Geometry: final body of the model. Coordinates: model frame, mm. A direction names the side the tool comes from. Give positions to 0.01 mm unless a question says otherwise; leave off trailing zeros. Order: outer loops, then holes, each group sorted by start corner. A loop starts at its lowest first (then second) coordinate and runs counter-clockwise, first axis right, second up. Notation, with made-up numbers: M 47,72.5 L 68,72.5 A9 cw 68,76.5 Z; hole C 13.25,21.25 d1. An arc over 180 degrees is marked long. One line per item, written item: value. Start each with the question number.
```python
from build123d import *

# Parameters (mm, degrees)
SKETCH1_R           = 40
BOSS_EXTRUDE1_DEPTH = 139
SKETCH2_R           = 40
SKETCH2_R_2         = 25
CUT_EXTRUDE1_DEPTH  = 19
CUT_EXTRUDE2_START  = -19
SKETCH3_R           = 40
SKETCH3_R_2         = 25
CUT_EXTRUDE2_DEPTH  = 19
FILLET1_R           = 2
CUT_EXTRUDE7_DEPTH  = 151.069983674
CUT_EXTRUDE8_DEPTH  = 151.069983674
CUT_EXTRUDE9_DEPTH  = 151.069983674
SKETCH8_R           = 3.75
CUT_EXTRUDE10_DEPTH = 151.069983674
CIRPATTERN1_COUNT   = 12
CUT_EXTRUDE14_DEPTH = 151.069983674


with BuildPart() as part:
    # Sketch1 → Boss-Extrude1 (new body)
    with BuildSketch(Plane.XY):
        Circle(SKETCH1_R)
    extrude(amount=-BOSS_EXTRUDE1_DEPTH)

    # Sketch2 → Cut-Extrude1 (cut)
    with BuildSketch(Plane.XY):
        Circle(SKETCH2_R)
        Circle(SKETCH2_R_2, mode=Mode.SUBTRACT)
    extrude(amount=-CUT_EXTRUDE1_DEPTH, mode=Mode.SUBTRACT)

    # Sketch3 → Cut-Extrude2 (cut)
    with BuildSketch(Plane(origin=(0, 0, -139), x_dir=(-1, 0, 0), z_dir=(0, 0, -1)).offset(CUT_EXTRUDE2_START)):
        with Locations(Location((0, 0, 0), (0, 0, 180))):
            Circle(SKETCH3_R)
        with Locations(Location((0, 0, 0), (0, 0, 180))):
            Circle(SKETCH3_R_2, mode=Mode.SUBTRACT)
    extrude(amount=CUT_EXTRUDE2_DEPTH, mode=Mode.SUBTRACT)

    # Fillet1
    fillet1_edges = [part.edges().sort_by_distance(p)[0] for p in [
        (-25, 0, -120),
        (-25, 0, -19),
    ]]
    fillet(fillet1_edges, radius=FILLET1_R)

    # Sketch5 → Cut-Extrude7 (cut, through all)
    with BuildSketch(Plane.XY):
        Polygon((0, 40), (0, 0), (40, 0), align=None)
    extrude(amount=-CUT_EXTRUDE7_DEPTH, mode=Mode.SUBTRACT)


with BuildPart() as body_2:
    # of the pieces the cut leaves, the one that is kept (cut_extrude7_keep)
    add(part.part.solids().sort_by_distance((27, 0, -120))[0])

    # Sketch6 → Cut-Extrude8 (cut, through all)
    with BuildSketch(Plane.XY):
        with BuildLine():
            Line((12, 4), (-12, 4))
            ThreePointArc((-12, 4), (-15, 7), (-12, 10))
            Line((-12, 10), (12, 10))
            ThreePointArc((12, 10), (15, 7), (12, 4))
        make_face()
    extrude(amount=-CUT_EXTRUDE8_DEPTH, mode=Mode.SUBTRACT)

    # Sketch7 → Cut-Extrude9 (cut, through all)
    with BuildSketch(Plane(origin=(0, 0, 0), x_dir=(0, 0, -1), z_dir=(1, 0, 0))):
        Polygon((91.5, 40), (47.5, 40), (50, 37.5), (89, 37.5), align=None)
    extrude(amount=-CUT_EXTRUDE9_DEPTH, mode=Mode.SUBTRACT)

    # Sketch8 → Cut-Extrude10 (cut, through all)
    with BuildSketch(Plane.XY):
        with Locations((-8.282209443, 30.909626441)):
            Circle(SKETCH8_R)
    cut_extrude10 = extrude(amount=-CUT_EXTRUDE10_DEPTH, mode=Mode.SUBTRACT)

    # CirPattern1: Cut-Extrude10 ×12 about axis
    cirpattern1_axis = Axis((0, 0, -19), (0, 0, 1))
    for i in range(1, CIRPATTERN1_COUNT):
        add(cut_extrude10.rotate(cirpattern1_axis, i * 360 / CIRPATTERN1_COUNT), mode=Mode.SUBTRACT)

    # Sketch9 → Cut-Extrude14 (cut, through all)
    with BuildSketch(Plane(origin=(0, 0, 0), x_dir=(1, 0, 0), z_dir=(0, 1, 0))):
        with BuildLine():
            Line((40, 139), (10, 139))
            ThreePointArc((10, 139), (10.114159057, 136.385327718), (10.45576741, 133.79055467))
            Line((10.45576741, 133.79055467), (40, 139))
        make_face()
        with BuildLine():
            Line((40, 109), (40, 139))
            Line((40, 139), (27.321452148, 111.810766389))
            ThreePointArc((27.321452148, 111.810766389), (33.506811582, 109.711119786), (40, 109))
        make_face()
        with BuildLine():
            Line((27.321452148, 111.810766389), (40, 139))
            Line((40, 139), (10.45576741, 133.79055467))
            ThreePointArc((10.45576741, 133.79055467), (16.199399791, 120.73715713), (27.321452148, 111.810766389))
        make_face()
        with BuildLine():
            ThreePointArc((27.321452148, 111.810766389), (16.199399791, 120.73715713), (10.45576741, 133.79055467))
            Line((10.45576741, 133.79055467), (5.531728645, 132.922313782))
            ThreePointArc((5.531728645, 132.922313782), (12.23263309, 117.693349985), (25.208360839, 107.279227454))
            Line((25.208360839, 107.279227454), (27.321452148, 111.810766389))
        make_face()
    extrude(amount=-CUT_EXTRUDE14_DEPTH, mode=Mode.SUBTRACT)


solid = body_2.part
```
Q1. Set-up query: faces 1 (the face through (0, 25, -69)), 2 (the face through (-6, -5, 0)), 3 (the face through (26.25, -15.31, -109.51)), 4 (the face through (12, -15, -118)), 5 (the face through (-6, 4, -69)). Return all of +Z, -Z, +X, -X, +Y, -Y with unobstructed straight access to the full face (end or side cutting, diameter ignored); none if empty.
Q2. Section query C-C on z = -125. Return loops of the section in (x, y), and give its area (3 significant figures).
Q3. Contact query for flat-ended pins moving along their axis: pin 1 (3.5 mm diameter, centred on x = -3, z = -67.5, fed in from -Y); pin 2 (12 mm diameter, centred on x = 30.91, y = -8.28, fed in from -Z); pin 3 (10 mm diameter, centred on x = -22.63, y = -22.63, fed in from -Z). Output: stop coordinate, or through.
Q4. Section query B-B on z = -94. Give the number of separate pieces and of enclosed holes in the cut face, and give its area (3 significant figures).
Q5. Section query A-A on x = 32. Return loops of the section in (y, z).
Q6. Ray query, line 1 along Y through (x, z) = (-8, -102.5); line 2 along Y through (x, z) = (-32, -115.5); line 3 along Y through (x, z) = (-23.5, -31). Return the intervals inside material, ascending. Write a range as [from, to].
Q7. Mould query, pull axis Z, two halves, no side actions, for faces 6 (the face through (-9.718, -34.374, -68.793)), 7 (the face through (34.844, -11.157, -109.446)), 8 (the face through (-7, 37.5, -69)). Classes: +Z half, -Z half, draft (parallel to the pull), parting line (faces both ways), or undercut.
Results below:
1. face 1: +Z, -Z, +X, +Y
1. face 2: +Z, +X, -X, +Y, -Y
1. face 3: -Z, +Y, -Y
1. face 4: +Y, -Y
1. face 5: +Z, -Z, +X
2. outline: M -12,4 A3 cw -12,10 L 0,10 L 0,25 A25 ccw long 7.92,-23.71 L 7.92,0 L 0,0 L 0,4 Z
2. area: 1,090 mm2
3. pin 1: y = -39.98
3. pin 2: z = -111.81
3. pin 3: z = -120
4. separate pieces: 1
4. enclosed holes: 9
4. area: 3,290 mm2
5. outline: M -24,-110.09 L -11.87,-110.09 L -11.87,-19 L -24,-19 Z; M -4.69,-110.09 L 0,-110.09 L 0,-19 L -4.69,-19 Z
6. line 1: [-39.19, -34.65], [-27.17, 4], [10, 27.17], [34.65, 39.19]
6. line 2: [-24, -11.87], [-4.69, 4.69], [11.87, 24]
6. line 3: [-32.37, -26.27], [-18.98, 18.98], [26.27, 32.37]
7. face 6: draft
7. face 7: -Z half
7. face 8: undercut
